Can you work these out from the drawing? Everything is in mm from the part's minimum corner. Give positions to 0.01 mm unless a question says otherwise; leave off trailing zeros. Write each loop counter-clockwise with the first axis right and the second up, starting at its lowest first coordinate (ties: lowest second). Pieces come first, ordered by that corner, then holes. Notation, with made-up numbers: (36, 42.25) - (64, 42.25) arc R15 cw to (64, 58.25) - close; hole circle Ø8 at (-24.5, 12). An arc over 180 degrees is marked (long way). Answer in a Markdown table with one row per item.
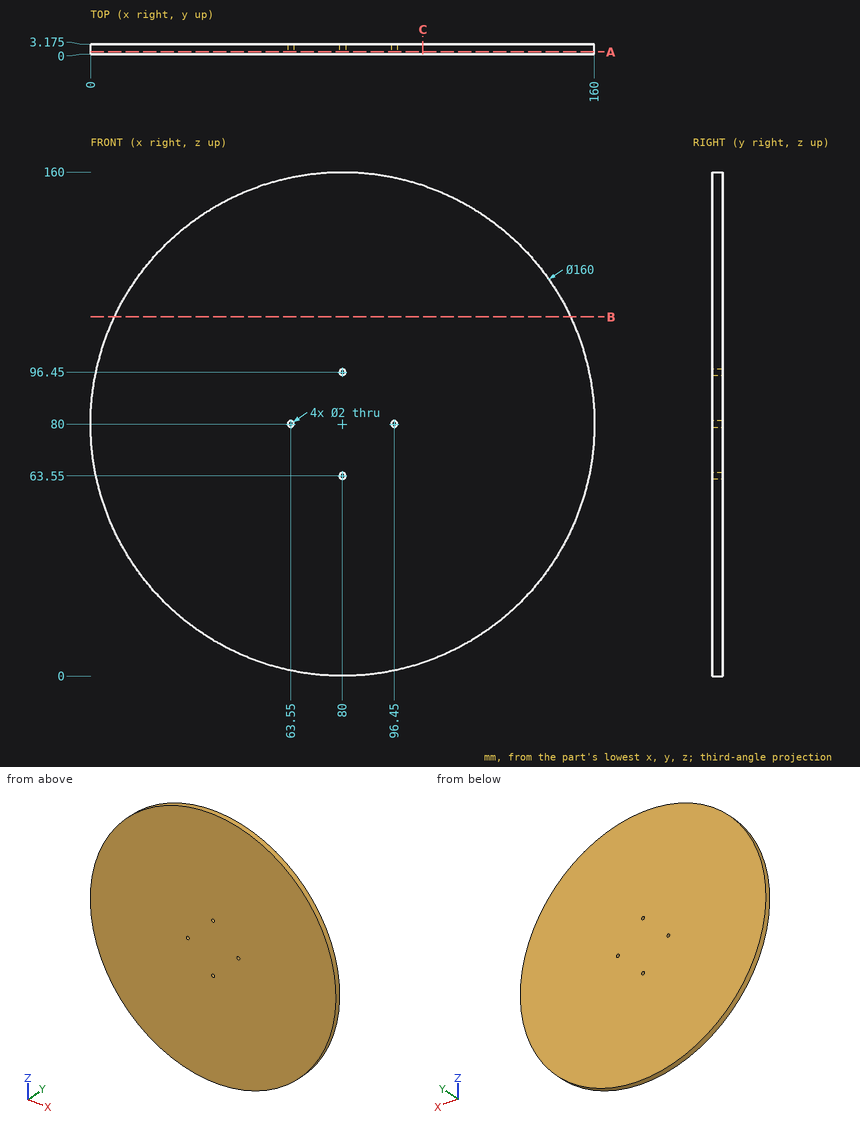
1) Imagine slicing it at C-C (x = 105.5). List the corners of the cut face in (y, z) for me (3 decimals).
Check values:
| item | result |
|---|---|
| outline | (0, 4.173) - (3.175, 4.173) - (3.175, 155.827) - (0, 155.827) - close |
2) Imagine slicing it at B-B (z = 114). List the corners of the cut face in (x, y) for me (3 decimals), then the cut area to 3 significant figures.
Check values:
| item | result |
|---|---|
| outline | (7.585, 0) - (152.415, 0) - (152.415, 3.175) - (7.585, 3.175) - close |
| area | 460 mm2 |
3) Will these pins go through, and if not, where does the flat tip stop? P1, Ø1, axis at x = 22.5, y = 1.5, coming from the +Z side; P2, Ø1.5, axis at x = 97, y = 1, coming from the -Z side.
Check values:
| item | result |
|---|---|
| P1 | stops at z = 136.13 |
| P2 | stops at z = 1.67 |
4) If I drill on line 1 (X direction, y = 2.2, z = 80); line 2 (Z direction, x = 80.5, y = 2.2); line 3 (X direction, y = 2.5, z = 96.45), over which ranges is the centre line in solid material (lowest first)?
Check values:
| item | result |
|---|---|
| line 1 | x = 0 to 62.55, 64.55 to 95.45, 97.45 to 160 |
| line 2 | z = 0 to 62.68, 64.42 to 95.58, 97.32 to 160 |
| line 3 | x = 1.71 to 79, 81 to 158.29 |
5) Imagine slicing it at A-A (y = 0.7). List the corners of the cut face in (x, z) for me, then the cut area to 3 significant figures.
Check values:
| item | result |
|---|---|
| outline | circle Ø160 at (80, 80); hole circle Ø2 at (63.55, 80); hole circle Ø2 at (80, 63.55); hole circle Ø2 at (80, 96.45); hole circle Ø2 at (96.45, 80) |
| area | 20,100 mm2 |
